Input: part model. Units: mm. Frame: model coordinates. A direction names the side the tool comes from. Round coordinates to 2 decimals unless told otherwise and drop trailing zeros. Write each loop counter-clockwise with the first axis right and the second up, starting at its lowest first coordinate (ties: lowest second). Pieces come first, ordered by that corner, then holes. Notation, with made-up numbers: M 80.5,53.25 L 100.5,53.25 A21 cw 100.5,79.25 Z; hole C -10.5,19.25 d8. An arc over 180 degrees is marked long. Write each question's results on one line, items separated by ' | '. Start each with the question number.
```python
from build123d import *

# Parameters (mm, degrees)
SKETCH_1_R               = 6
EXTRUDE_1_DEPTH          = 2
SKETCH_1_3_R             = 6
SKETCH_1_3_R_2           = 3.5
EXTRUDE_2_DEPTH          = 11
RIB_1_REACH              = 40.293
SKETCH_2_WALL_W          = 84.606091636
SKETCH_2_WALL_H          = 3
PATTERN_CIRCULAR_1_COUNT = 2


with BuildPart() as part:
    # Sketch 1 → Extrude 1 (new body)
    with BuildSketch(Plane.XY):
        with BuildLine():
            Line((30, 6.5), (0, 6.5))
            ThreePointArc((0, 6.5), (-3.716517187, 5.332682252), (-6.098155459, 2.25))
            Line((-6.098155459, 2.25), (0, 2.25))
            ThreePointArc((0, 2.25), (2.25, 0), (0, -2.25))
            Line((0, -2.25), (-6.098155459, -2.25))
            ThreePointArc((-6.098155459, -2.25), (-3.716517187, -5.332682252), (0, -6.5))
            Line((0, -6.5), (30, -6.5))
            ThreePointArc((30, -6.5), (33.716517187, -5.332682252), (36.098155459, -2.25))
            Line((36.098155459, -2.25), (30, -2.25))
            ThreePointArc((30, -2.25), (27.75, 0), (30, 2.25))
            Line((30, 2.25), (36.098155459, 2.25))
            ThreePointArc((36.098155459, 2.25), (33.716517187, 5.332682252), (30, 6.5))
        make_face()
        with Locations((15, 0)):
            Circle(SKETCH_1_R, mode=Mode.SUBTRACT)
    extrude(amount=EXTRUDE_1_DEPTH)

    # Sketch 1_3 → Extrude 2 (add)
    with BuildSketch(Plane.XY):
        with Locations(Location((15, 0, 0), (0, 0, 180))):
            Circle(SKETCH_1_3_R)
        with Locations(Location((15, 0, 0), (0, 0, 180))):
            Circle(SKETCH_1_3_R_2, mode=Mode.SUBTRACT)
    extrude(amount=EXTRUDE_2_DEPTH)

    # Sketch 2 wall → Rib 1 (add, up to next)
    with BuildSketch(Plane(origin=(7, 0, 4.25), x_dir=(0.66436383883, 0, 0.747409318684), z_dir=(0.747409318684, 0, -0.66436383883)), mode=Mode.PRIVATE) as rib_1_sk1:
        Rectangle(SKETCH_2_WALL_W, SKETCH_2_WALL_H)
    rib_1_tool1 = extrude(rib_1_sk1.sketch, amount=RIB_1_REACH, mode=Mode.PRIVATE) - part.part
    rib_1 = rib_1_tool1.solids().sort_by_distance((7, 0, 4.25))[0]
    add(rib_1)

    # Pattern Circular 1: Rib 1 ×2 about axis
    pattern_circular_1_axis = Axis((15, 0, 11), (0, 0, -1))
    for i in range(1, PATTERN_CIRCULAR_1_COUNT):
        add(rib_1.rotate(pattern_circular_1_axis, i * 360 / PATTERN_CIRCULAR_1_COUNT))


solid = part.part
```
1. Cut plane A-A on x = 15. Output: boundary loops of the cut face in (y, z), and give its area (3 significant figures).
2. Cut plane B-B on y = 0. Output: boundary loops of the cut face in (x, z).
3. Cut plane D-D on z = 3. Output: boundary loops of the cut face in (x, y).
4. Access query for faces 1 (the face through (9.277, -1.802, 6.437)), 2 (the face through (8, -1.5, 4)), 3 (the face through (33, -2.25, 1)), 4 (the face through (22, 1.5, 4)), 5 (the face through (8, 1.5, 4)). Directions: +Z, -Z, +X, -X, +Y, -Y. A direction counts if a zero-diameter tool reaches every point of the face in a straight line with its end or side. Return the directions, or none.
5. Contact query for flat-ended pins moving along their axis: P1, Ø1, axis at x = 33, z = 1.5, coming from the -Y side; P2, Ø2, axis at x = 31.5, z = 1, coming from the +Y side; P3, Ø0.6, axis at x = -2.5, z = 0.5, coming from the +Y side; P4, Ø4, axis at x = 13, y = 2, coming from the -Z side. Output: stop coordinate, or through.
6. Line query: L1, parallel to Y at x = 15, z = 3.75; L2, parallel to Y at x = 24.5, z = 2.5; L3, parallel to Z at x = 8.5, y = -4.75. Output: solid intervals per line, ascending. Write a range as from..to.
7. Cut plane C-C on x = 7. Output: boundary loops of the cut face in (y, z), and give its area (4 significant figures).
8. Draft query along X for faces 6 (the face through (11.66, -1.05, 5.42)), 7 (the face through (33.671, -5.364, 0.986)), 8 (the face through (-3, 2.25, 1)). Return one class per face: +X half, -X half, draft (parallel to the pull), parting line (faces both ways), or undercut.
Answers follow:
1) outline: M -6.5,0 L -3.5,0 L -3.5,11 L -6,11 L -6,2 L -6.5,2 Z; M 3.5,0 L 6.5,0 L 6.5,2 L 6,2 L 6,11 L 3.5,11 Z | area: 57.0 mm2
2) outline: M 2.25,0 L 11.5,0 L 11.5,11 L 9,11 L 9,6.5 L 5,2 L 2.25,2 Z; M 18.5,0 L 27.75,0 L 27.75,2 L 25,2 L 21,6.5 L 21,11 L 18.5,11 Z
3) outline: M 5.89,-1.5 L 9.19,-1.5 A6 ccw 20.81,-1.5 L 24.11,-1.5 L 24.11,1.5 L 20.81,1.5 A6 ccw 9.19,1.5 L 5.89,1.5 Z; hole C 15,0 d7
4) face 1: +Z | face 2: +Z, -X, -Y | face 3: +Z, -Z, +X | face 4: +Z, +X, +Y | face 5: +Z, -X, +Y
5) P1: stops at y = -6 | P2: stops at y = 6.48 | P3: stops at y = 6.12 | P4: stops at z = 0
6) L1: y = -6..-3.5, 3.5..6 | L2: y = -1.5..1.5 | L3: z = 0..2
7) outline: M -6.5,0 L 6.5,0 L 6.5,2 L 1.5,2 L 1.5,4.25 L -1.5,4.25 L -1.5,2 L -6.5,2 Z | area: 32.75 mm2
8) face 6: undercut | face 7: +X half | face 8: draft
